CAD build for the part. Positions are in the model's coordinates, mm. Face numbers are marked on the shaded views. A direction names the side the tool comes from. Round coordinates to 2 decimals unless told otherwise and drop trailing zeros. Loops run counter-clockwise (first coordinate to the right, second up) from the corner with the lowest first, then second, coordinate; pieces in that order, holes last.
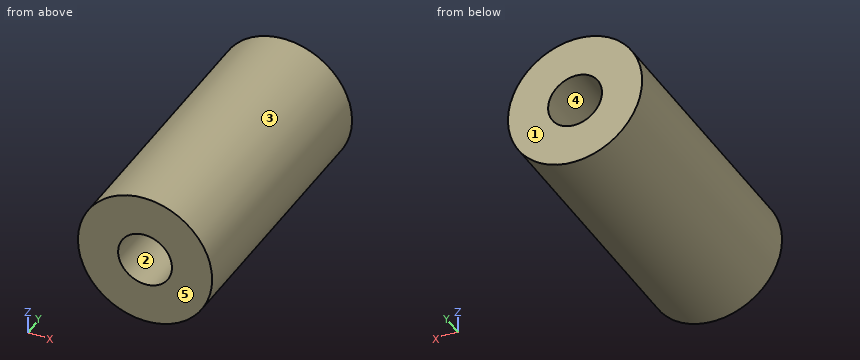
```python
from build123d import *

# Parameters (mm, degrees)
SKETCH1_R                = 8.35
SKETCH1_R_2              = 3.35
BOSS_EXTRUDE1_DEPTH      = 34
BOSS_EXTRUDE2_DEPTH      = 0.5
BOSS_EXTRUDE2_DEPTH_BACK = 0.5
SKETCH2_R                = 3.35
SKETCH2_R_2              = 2.35
CHAMFER1_SIZE            = 1


with BuildPart() as part:
    # Sketch1 → Boss-Extrude1 (new body)
    with BuildSketch(Plane(origin=(0, 0, 0), x_dir=(1, 0, 0), z_dir=(0, 1, 0))):
        with Locations(Location((0, 0, 0), (0, 0, 270))):
            Circle(SKETCH1_R)
        with Locations(Location((0, 0, 0), (0, 0, 270))):
            Circle(SKETCH1_R_2, mode=Mode.SUBTRACT)
    extrude(amount=BOSS_EXTRUDE1_DEPTH)

    # Sketch2 → Boss-Extrude2 (add, two sides: drawn at the far end of the back side and taken through both)
    with BuildSketch(Plane(origin=(0, 17, 0), x_dir=(1, 0, 0), z_dir=(0, 1, 0)).offset(-BOSS_EXTRUDE2_DEPTH_BACK)):
        with Locations(Location((0, 0, 0), (0, 0, 270))):
            Circle(SKETCH2_R)
        with Locations(Location((0, 0, 0), (0, 0, 270))):
            Circle(SKETCH2_R_2, mode=Mode.SUBTRACT)
    extrude(amount=BOSS_EXTRUDE2_DEPTH + BOSS_EXTRUDE2_DEPTH_BACK)

    # Chamfer1
    chamfer1_edges = [part.edges().sort_by_distance(p)[0] for p in [
        (0, 17.5, -3.35),
        (0, 16.5, -3.35),
    ]]
    chamfer(chamfer1_edges, length=CHAMFER1_SIZE - 0.0001)  # a hair under: the kernel refuses the full size


solid = part.part
```
Item 1: Two-plate mould, pull along X, no slides. Class the marked faces 3, 4 and 5: released by +X, released by -X, zero draft, split by the parting line, or undercut.
Answers follow:
face 3: split by the parting line
face 4: undercut
face 5: zero draft
Item 2: Probe line 1 (X direction, y = 16.8, z = 0); line 2 (X direction, y = 11.25, z = 0); line 3 (Z direction, x = 1.25, y = 21). List the from-to ranges inside material, lowest first.
Answers follow:
line 1: x = -8.35 to -2.35, 2.35 to 8.35
line 2: x = -8.35 to -3.35, 3.35 to 8.35
line 3: z = -8.26 to -3.11, 3.11 to 8.26
Item 3: Flat gauge pins, fed straight in: P1, Ø5, axis at x = -0.5, z = 0, coming from the +Y side; P2, Ø6, axis at x = 0, z = 0, coming from the -Y side; P3, Ø4, axis at x = -1, z = 0.5, coming from the -Y side. Where does each tip first touch, or does it go through?
Answers follow:
P1: stops at y = 18.15
P2: stops at y = 15.85
P3: stops at y = 15.73
Item 4: Cut at D-D, the plane x = 4.5. Give the cut face in (y, z).
Answers follow:
outline: (0, -7.03) - (34, -7.03) - (34, 7.03) - (0, 7.03) - close
Item 5: 3-axis set-ups, long thin cutter, end or side, ignore diameter. For the marked faces 1 and 2: which of +Z, -Z, +X, -X, +Y, -Y reach the whole face in a straight line?
Answers follow:
face 1: +Z, -Z, +X, -X, +Y
face 2: -Y
Item 6: Cut at C-C, the plane y = 12. Give the cut face in (x, z).
Answers follow:
outline: circle Ø16.7 at (0, 0); hole circle Ø6.7 at (0, 0)
